```python
from build123d import *

# Parameters (mm, degrees)
F0_R     = 1.55
F0_R_2   = 14.25
F0_R_3   = 1.2
F0_W     = 12
F0_H     = 2
F1_DEPTH = 1.2
F2_R     = 2


with BuildPart() as f1:
    # F0 (on Top) → F1 (new body)
    with BuildSketch(Plane.XY):
        Polygon((12.5, -15), (15, -15), (15, 15), (-15, 15), (-15, -15), (-12.5, -15), (-6, -15), (6, -15), align=None)
        with Locations((-12, -12)):
            Circle(F0_R, mode=Mode.SUBTRACT)
        with Locations((12, -12)):
            Circle(F0_R, mode=Mode.SUBTRACT)
        with Locations((-12, 12)):
            Circle(F0_R, mode=Mode.SUBTRACT)
        Circle(F0_R_2, mode=Mode.SUBTRACT)
        with Locations((12, 12)):
            Circle(F0_R, mode=Mode.SUBTRACT)
        Polygon((-6, -17), (-6, -15), (-12.5, -15), (-12.5, -20), (-6, -20), align=None)
        with Locations((-9.2, -18)):
            Circle(F0_R_3, mode=Mode.SUBTRACT)
        with Locations((0, -16)):
            Rectangle(F0_W, F0_H)
        Polygon((12.5, -20), (12.5, -15), (6, -15), (6, -17), (6, -20), align=None)
        with Locations((9.2, -18)):
            Circle(F0_R_3, mode=Mode.SUBTRACT)
    extrude(amount=F1_DEPTH)

    # F2
    f2_edges = [f1.edges().sort_by_distance(p)[0] for p in [
        (15, -15, 0.6),
        (-15, -15, 0.6),
        (-15, 15, 0.6),
        (15, 15, 0.6),
        (-12.5, -20, 0.6),
        (-6, -20, 0.6),
        (6, -20, 0.6),
        (12.5, -20, 0.6),
    ]]
    fillet(f2_edges, radius=F2_R)


solid = f1.part
```
Verification items for the finished model (mm, model axes). A direction names the side the tool comes from. Coordinates: 2 decimals unless noted, no trailing zeros. Loops run counter-clockwise (first coordinate to the right, second up) from the corner with the lowest first, then second, coordinate; pieces in that order, holes last. Notation, with made-up numbers: (48.25, 16) -> (59.25, 16) arc R14 cw to (59.25, 20) -> close; hole circle Ø1 at (58, 0). An arc over 180 degrees is marked (long way). Answer in a Markdown table with one row per item. Add a question column.
1. Section check D-D, the plane y = 11.5. Enter the section's corners in (x, z).
2. Access from +Z, -Z, +X, -X, +Y, -Y to the whole of each face (thin tool, end or side, straight path). Record for faces 5 (the face through (-6.6, -19.43, 0.61)), 6 (the face through (-15, 0, 1)).
3. Section check B-B, the plane x = 9.2. Enter the section's corners in (y, z).
4. Material ranges on probe 1 along Y at (x, z) = (-8.5, 1.05); probe 2 along X at (y, z) = (-17.5, 0.35); probe 3 along X at (y, z) = (-13, 0.45), recorded low to high. Write a range as [from, to].
5. Section check A-A, the plane y = 0. Enter the section's corners in (x, z), then the cut area to 3 significant figures.
6. Depth check by flat-ended pin: P1, Ø2.5, axis at x = 12, y = 12, coming from the -Z side; P2, Ø0.6, axis at x = -12.5, z = 0.5, coming from the -Y side; P3, Ø0.5, axis at y = -17.5, z = 0.5, coming from the +X side. Enter the tip coordinate at first touch or a pass-through.
7. Draft check along X on faces 1 (the face through (14.43, -14.4, 0.61)), 2 (the face through (13.163, -5.458, 0.592)), 3 (the face through (-12.5, -16, 1)), 4 (the face through (-13.23, 11.06, 0.59)). Enter one of: +X half, -X half, draft (parallel to the pull), parting line (faces both ways), or undercut.
8. Section check C-C, the plane z = 1. Enter the section's corners in (x, y).
Derived:
| question | item | result |
|---|---|---|
| 1 | outline | (-15, 0) -> (-13.47, 0) -> (-13.47, 1.2) -> (-15, 1.2) -> close; (-10.53, 0) -> (-8.42, 0) -> (-8.42, 1.2) -> (-10.53, 1.2) -> close; (8.42, 0) -> (10.53, 0) -> (10.53, 1.2) -> (8.42, 1.2) -> close; (13.47, 0) -> (15, 0) -> (15, 1.2) -> (13.47, 1.2) -> close |
| 2 | face 5 | +Z, -Z, -Y |
| 2 | face 6 | +Z, -Z, -X, +Y, -Y |
| 3 | outline | (-20, 0) -> (-19.2, 0) -> (-19.2, 1.2) -> (-20, 1.2) -> close; (-16.8, 0) -> (-10.88, 0) -> (-10.88, 1.2) -> (-16.8, 1.2) -> close; (10.88, 0) -> (15, 0) -> (15, 1.2) -> (10.88, 1.2) -> close |
| 4 | probe 1 | y = [-20, -18.97], [-17.03, -11.44], [11.44, 15] |
| 4 | probe 2 | x = [-12.5, -10.29], [-8.11, -6], [6, 8.11], [10.29, 12.5] |
| 4 | probe 3 | x = [-15, -13.18], [-10.82, -5.84], [5.84, 10.82], [13.18, 15] |
| 5 | outline | (-15, 0) -> (-14.25, 0) -> (-14.25, 1.2) -> (-15, 1.2) -> close; (14.25, 0) -> (15, 0) -> (15, 1.2) -> (14.25, 1.2) -> close |
| 5 | area | 1.80 mm² |
| 6 | P1 | passes through |
| 6 | P2 | stops at y = -19.05 |
| 6 | P3 | stops at x = 12.5 |
| 7 | face 1 | +X half |
| 7 | face 2 | undercut |
| 7 | face 3 | -X half |
| 7 | face 4 | undercut |
| 8 | outline | (-15, -13) arc R2 ccw to (-13, -15) -> (-12.5, -15) -> (-12.5, -18) arc R2 ccw to (-10.5, -20) -> (-8, -20) arc R2 ccw to (-6, -18) -> (-6, -17) -> (6, -17) -> (6, -18) arc R2 ccw to (8, -20) -> (10.5, -20) arc R2 ccw to (12.5, -18) -> (12.5, -15) -> (13, -15) arc R2 ccw to (15, -13) -> (15, 13) arc R2 ccw to (13, 15) -> (-13, 15) arc R2 ccw to (-15, 13) -> close; hole circle Ø28.5 at (0, 0); hole circle Ø3.1 at (-12, -12); hole circle Ø3.1 at (-12, 12); hole circle Ø2.4 at (-9.2, -18); hole circle Ø2.4 at (9.2, -18); hole circle Ø3.1 at (12, -12); hole circle Ø3.1 at (12, 12) |
